Can you work these out from the drawing? Everything is in mm from the part's minimum corner. Round coordinates to 2 decimals unless told otherwise and drop trailing zeros. Use a Markdown table: item, result. Add a question column.
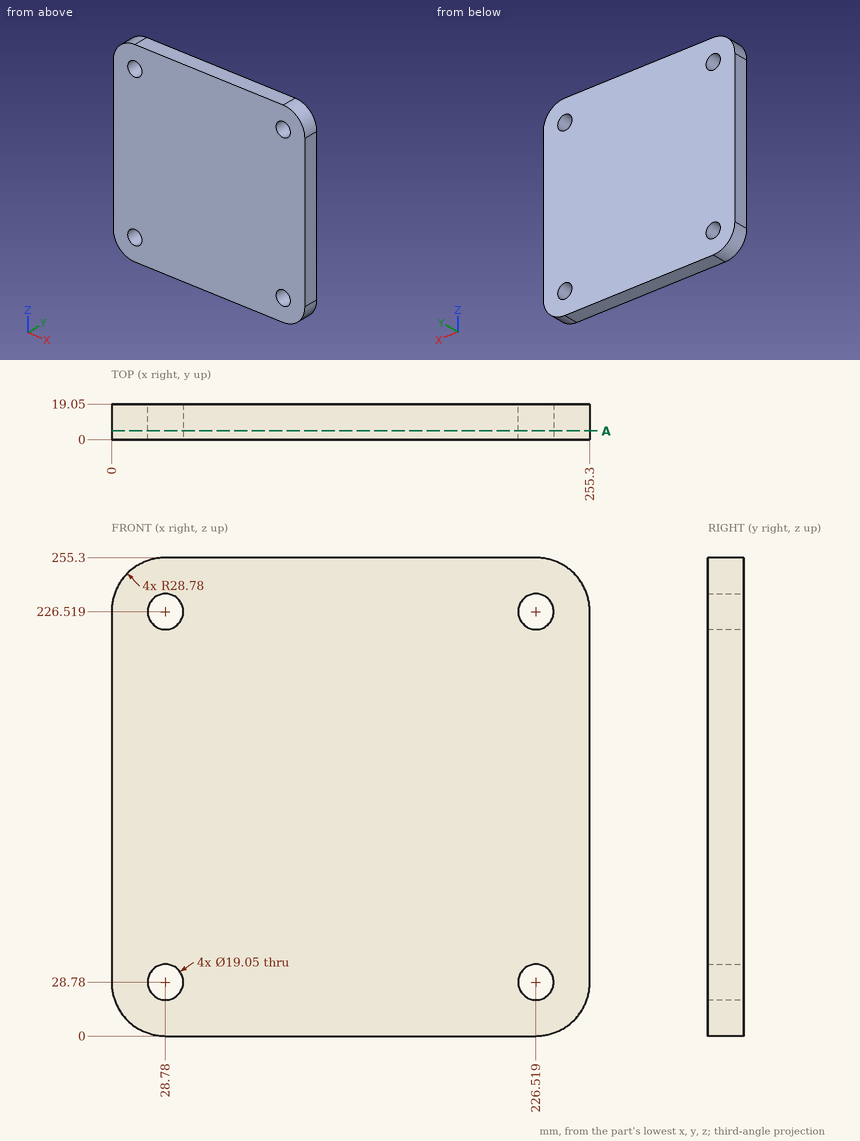
Item 1: For pin 1 Ø17 at (x, z) = (28.78, 28.78) entering from +Y, with a flat end and sliding along its axis, tell me the tip position at first contact or that it passes through.
Item 2: Imagine slicing it at A-A on y = 4.75. Count the separate pieces of the cut face and the enclosed holes in it, plus the area to 3 significant figures.
Item 3: I need wall thicknesses on probe 1 along Z at (x, y) = (229.5, 1.75) (1 decimal); probe 2 along Z at (x, y) = (36.5, 9.75); probe 3 along X at (y, z) = (12.25, 222.5) (1 decimal). Which ranges of each line are inside material? Lowest first, please. Write a range as from..to.
The answers:
| question | item | result |
|---|---|---|
| 1 | pin 1 | through |
| 2 | separate pieces | 1 |
| 2 | enclosed holes | 4 |
| 2 | area | 63,300 mm² |
| 3 | probe 1 | 0.2..19.7, 37.8..217.5, 235.6..255.1 |
| 3 | probe 2 | 0..23.2, 34.36..220.94, 232.1..255.3 |
| 3 | probe 3 | 0..20.1, 37.4..217.9, 235.2..255.3 |
